```python
from build123d import *

# Parameters (mm, degrees)
F1_DEPTH = 5


with BuildPart() as f1:
    # F0 (on Top) → F1 (new body)
    with BuildSketch(Plane.XY):
        with BuildLine():
            add(Edge.make_bspline(
                [(42.347362, 79.562907), (42.134291, 81.886016), (41.708148, 86.532233), (41.068935, 93.501559), (40.642792, 98.147776), (40.429721, 100.470884)],
                knots=[0, 0, 0, 0, 6.998578, 13.997156, 20.995734, 20.995734, 20.995734, 20.995734], degree=3))
            ThreePointArc((40.429721, 100.470884), (37.441749, 108.15842), (30.429721, 112.50096))
            ThreePointArc((30.429721, 112.50096), (22.730822, 113.923703), (14.929721, 114.587078))
            ThreePointArc((14.929721, 114.587078), (4.429721, 114.770884), (-6.070279, 114.587078))
            ThreePointArc((-6.070279, 114.587078), (-13.87138, 113.923703), (-21.570279, 112.50096))
            ThreePointArc((-21.570279, 112.50096), (-28.582306, 108.15842), (-31.570279, 100.470884))
            add(Edge.make_bspline(
                [(-31.570279, 100.470884), (-31.78335, 98.147776), (-32.209492, 93.501559), (-32.848706, 86.532233), (-33.274848, 81.886016), (-33.487919, 79.562907)],
                knots=[0, 0, 0, 0, 6.998578, 13.997156, 20.995734, 20.995734, 20.995734, 20.995734], degree=3))
            ThreePointArc((-33.487919, 79.562907), (-33.026295, 77.670215), (-31.499503, 76.460138))
            add(Edge.make_bspline(
                [(-31.499503, 76.460138), (-29.46591, 75.741927), (-25.398724, 74.305504), (-19.297945, 72.15087), (-15.230758, 70.714447), (-13.197165, 69.996235)],
                knots=[0, 0, 0, 0, 6.470082, 12.940164, 19.410245, 19.410245, 19.410245, 19.410245], degree=3))
            ThreePointArc((-13.197165, 69.996235), (-10.571416, 68.677315), (-8.718314, 66.396937))
            ThreePointArc((-8.718314, 66.396937), (-7.368697, 63.253483), (-6.440564, 59.960864))
            ThreePointArc((-6.440564, 59.960864), (-4.477148, 47.55951), (-3.820279, 35.020884))
            add(Edge.make_bspline(
                [(-3.820279, 35.020884), (-3.820279, 31.465329), (-3.820279, 24.354218), (-3.820279, 13.687551), (-3.820279, 6.57644), (-3.820279, 3.020884)],
                knots=[0, 0, 0, 0, 10.666667, 21.333333, 32, 32, 32, 32], degree=3))
            ThreePointArc((-3.820279, 3.020884), (-4.477148, -9.517741), (-6.440564, -21.919096))
            ThreePointArc((-6.440564, -21.919096), (-7.368697, -25.211715), (-8.718314, -28.355168))
            ThreePointArc((-8.718314, -28.355168), (-10.571416, -30.635546), (-13.197165, -31.954467))
            add(Edge.make_bspline(
                [(-13.197165, -31.954467), (-16.443947, -33.101144), (-22.93751, -35.394499), (-32.677854, -38.834532), (-39.171417, -41.127887), (-42.418199, -42.274564)],
                knots=[0, 0, 0, 0, 10.329963, 20.659926, 30.989889, 30.989889, 30.989889, 30.989889], degree=3))
            ThreePointArc((-42.418199, -42.274564), (-47.569185, -43.714534), (-52.866234, -44.454425))
            add(Edge.make_bspline(
                [(-52.866234, -44.454425), (-54.420823, -44.566355), (-57.530001, -44.790216), (-62.193768, -45.126007), (-65.302946, -45.349868), (-66.857535, -45.461798)],
                knots=[0, 0, 0, 0, 4.67584, 9.35168, 14.027519, 14.027519, 14.027519, 14.027519], degree=3))
            ThreePointArc((-66.857535, -45.461798), (-69.498506, -46.726496), (-70.570279, -49.45147))
            add(Edge.make_bspline(
                [(-70.570279, -49.45147), (-70.570279, -50.093431), (-70.570279, -51.377352), (-70.570279, -53.303234), (-70.570279, -54.587155), (-70.570279, -55.229116)],
                knots=[0, 0, 0, 0, 1.925882, 3.851764, 5.777645, 5.777645, 5.777645, 5.777645], degree=3))
            ThreePointArc((-70.570279, -55.229116), (-69.984492, -56.643329), (-68.570279, -57.229116))
            add(Edge.make_bspline(
                [(-68.570279, -57.229116), (-60.459168, -57.229116), (-44.236945, -57.229116), (-19.903612, -57.229116), (-3.68139, -57.229116), (4.429721, -57.229116)],
                knots=[0, 0, 0, 0, 24.333333, 48.666667, 73, 73, 73, 73], degree=3))
            add(Edge.make_bspline(
                [(4.429721, -57.229116), (12.540832, -57.229116), (28.763055, -57.229116), (53.096388, -57.229116), (69.31861, -57.229116), (77.429721, -57.229116)],
                knots=[0, 0, 0, 0, 24.333333, 48.666667, 73, 73, 73, 73], degree=3))
            ThreePointArc((77.429721, -57.229116), (78.843935, -56.643329), (79.429721, -55.229116))
            add(Edge.make_bspline(
                [(79.429721, -55.229116), (79.429721, -54.587155), (79.429721, -53.303234), (79.429721, -51.377352), (79.429721, -50.093431), (79.429721, -49.45147)],
                knots=[0, 0, 0, 0, 1.925882, 3.851764, 5.777645, 5.777645, 5.777645, 5.777645], degree=3))
            ThreePointArc((79.429721, -49.45147), (78.357948, -46.726496), (75.716978, -45.461798))
            add(Edge.make_bspline(
                [(75.716978, -45.461798), (74.162389, -45.349868), (71.053211, -45.126007), (66.389444, -44.790216), (63.280266, -44.566355), (61.725677, -44.454425)],
                knots=[0, 0, 0, 0, 4.67584, 9.35168, 14.027519, 14.027519, 14.027519, 14.027519], degree=3))
            ThreePointArc((61.725677, -44.454425), (56.428627, -43.714534), (51.277641, -42.274564))
            add(Edge.make_bspline(
                [(51.277641, -42.274564), (48.03086, -41.127887), (41.537297, -38.834532), (31.796952, -35.394499), (25.303389, -33.101144), (22.056608, -31.954467)],
                knots=[0, 0, 0, 0, 10.329963, 20.659926, 30.989889, 30.989889, 30.989889, 30.989889], degree=3))
            ThreePointArc((22.056608, -31.954467), (19.430859, -30.635546), (17.577757, -28.355168))
            ThreePointArc((17.577757, -28.355168), (16.228139, -25.211715), (15.300007, -21.919096))
            ThreePointArc((15.300007, -21.919096), (13.33659, -9.517741), (12.679721, 3.020884))
            add(Edge.make_bspline(
                [(12.679721, 3.020884), (12.679721, 6.57644), (12.679721, 13.687551), (12.679721, 24.354218), (12.679721, 31.465329), (12.679721, 35.020884)],
                knots=[0, 0, 0, 0, 10.666667, 21.333333, 32, 32, 32, 32], degree=3))
            ThreePointArc((12.679721, 35.020884), (13.33659, 47.55951), (15.300007, 59.960864))
            ThreePointArc((15.300007, 59.960864), (16.228139, 63.253483), (17.577757, 66.396937))
            ThreePointArc((17.577757, 66.396937), (19.430859, 68.677315), (22.056608, 69.996235))
            add(Edge.make_bspline(
                [(22.056608, 69.996235), (24.090201, 70.714447), (28.157387, 72.15087), (34.258167, 74.305504), (38.325353, 75.741927), (40.358946, 76.460138)],
                knots=[0, 0, 0, 0, 6.470082, 12.940164, 19.410245, 19.410245, 19.410245, 19.410245], degree=3))
            ThreePointArc((40.358946, 76.460138), (41.885738, 77.670215), (42.347362, 79.562907))
        make_face()
    extrude(amount=F1_DEPTH)


solid = f1.part
```
Here's how the part is built. I have some questions about the finished solid (model axes, mm). A direction names the side the tool comes from. Give positions to 0.01 mm unless a question says otherwise; leave off trailing zeros. Loops run counter-clockwise (first coordinate to the right, second up) from the corner with the lowest first, then second, coordinate; pieces in that order, holes last. Notation, with made-up numbers: M 79.5,52 L 101.5,52 A20 ccw 101.5,82 Z; hole C 82,-5.5 d4. An arc over 180 degrees is marked long. Use one line per item in the form item = value. Start each with the question number.
Q1. Which directions (+Z, -Z, +X, -X, +Y, -Y) give clear straight access to the entire face, cutting with the end or side of a thin tool? Please do faces 1 (the cylindrical face through (-7.353, -25.167, 2.465)), 2 (the cylindrical face through (4.58, 114.77, 2.46)), 3 (the cylindrical face through (56.5, -43.73, 2.46)), 4 (the flat face through (-1, 16, 0)), 5 (the cylindrical face through (19.4, 68.65, 2.46)).
Q2. If we section it at A-A (y = -0.5): Write out the boundary of the cut face in (x, z).
Q3. If we section it at B-B (y = -18): Write out the boundary of the cut face in (x, z).
Q4. Thinking about a two-plate mould opening in Y: for faces 6 (the flat face through (-1, 16, 5)), 7 (the cylindrical face through (78.39, -46.76, 2.46)), 8 (the cylindrical face through (-4.496, 47.734, 2.465)), which applies, +Y half, -Y half, draft (parallel to the pull), parting line (faces both ways), or undercut?
Q5. I need wall thicknesses on line 1 along Y through (x, z) = (-21.5, 3.85); line 2 along X through (y, z) = (101, 3.5); line 3 along X through (y, z) = (101.5, 2.9). Which ranges of each line are inside material? Lowest first, please.
Taken from the geometry:
q1.face_1 = +Z, -Z, -X
q1.face_2 = +Z, -Z, +Y
q1.face_3 = +Z, -Z, +X, +Y
q1.face_4 = -Z, +X, -X, +Y, -Y
q1.face_5 = +Z, -Z, +X
q2.outline = M -3.87,0 L 12.73,0 L 12.73,5 L -3.87,5 Z
q3.outline = M -5.68,0 L 14.54,0 L 14.54,5 L -5.68,5 Z
q4.face_6 = draft
q4.face_7 = +Y half
q4.face_8 = undercut
q5.line_1 = -57.23 to -34.89, 72.93 to 112.52
q5.line_2 = -31.53 to 40.39
q5.line_3 = -31.48 to 40.34
